Here's how the part is built. I have some questions about the finished solid (model axes, mm). A direction names the side the tool comes from. Coordinates: 2 decimals unless noted, no trailing zeros. Order: outer loops, then holes, each group sorted by start corner. A loop starts at its lowest first (then second) coordinate and runs counter-clockwise, first axis right, second up. Notation, with made-up numbers: (-13.75, -1) - (28.25, -1) arc R14 ccw to (28.25, 4) - close; hole circle Ø4 at (87.5, 15.5). An arc over 180 degrees is marked (long way). Answer as CSV lines item,"result". Start each with the question number.
Q1. Suppose I cut it at A-A (z = 47). Please give me the cut outline in (x, y), then the cut area to 3 significant figures.
Q2. I need wall thicknesses on line 1 (X direction, y = 21.75, z = 51); line 2 (Y direction, x = -56, z = 15); line 3 (Z direction, x = -5, y = 11.75). Which ranges of each line are inside material? Lowest first, please.
Q3. Thinking about a two-plate mould opening in Z: for faces 3 (the face through (2, 12, 5)), 4 (the face through (-23, 25, 72)), 5 (the face through (-27, 7, 75)), 6 (the face through (-57.487, 10.564, 17.307)), which applies, released by +Z, released by -Z, zero draft, split by the parting line, or undercut?
Q4. For faces 1 (the face through (-57.49, 22.15, 8.01)), 2 (the face through (-28, 7, 70)), which set-ups out of +Z, -Z, +X, -X, +Y, -Y let a thin tool reach every point of the face, with its end or its side?
Q5. For pin 1 Ø8 at (x, y) = (-6, 20) entering from -Z; pin 2 Ø2 at (y, z) = (15, 12) entering from -X, each with a flat end and sliding along its axis, tell me the tip position at first contact or that it passes through.
Q6. Suppose I cut it at B-B (z = 18). Please give me the cut outline in (x, y).
Q7. Suppose I cut it at D-D (x = -44). Please give me the cut outline in (y, z).
Q8. Suppose I cut it at C-C (y = 3). Please give me the cut outline in (x, z).
Autodesk Inventor part; units mm, degrees
ref_plane "YZ Plane" through (0, 0, 0) normal (1, 0, 0) x (0, 1, 0)
ref_plane "XZ Plane" through (0, 0, 0) normal (0, 1, 0) x (-1, 0, 0)
ref_plane "XY Plane" through (0, 0, 0) normal (0, 0, 1) x (1, 0, 0)
sketch "Sketch1" plane through (0, 0, 0) normal (0, 1, 0) x (-1, 0, 0)
  line L0 (0.1515, 5) -> (-4.8485, 5)
  line L1 (-4.8485, 5) -> (-4.8485, 75)
  line L2 (-4.8485, 75) -> (0.1515, 75)
  line L3 (0.1515, 75) -> (0.1515, 5)
  line L4 (54.9515, 5) -> (54.9515, 58.2)
  line L5 (54.9515, 5) -> (59.9515, 5)
  line L6 (59.9515, 5) -> (59.9515, 75)
  line L7 (59.9515, 75) -> (54.9515, 75)
  line L8 (54.9515, 75) -> (54.9515, 5)
  line L9 (0.1515, 75) -> (54.9515, 75)
  line L10 (54.9515, 75) -> (54.9515, 70)
  line L11 (54.9515, 70) -> (0.1515, 70)
  line L12 (0.1515, 70) -> (0.1515, 75)
  point P0 (0, 0)
  point P1 (55.2, 35)
  dimension "d0" = 5
  dimension "d1" = 70
  dimension "d2" = 5
  dimension "d3" = 5
  dimension "d10" = 54.8
extrude "Extrusion1" add sketch "Sketch1" along normal blind 25
fillet "Fillet1" radius 10 4 edges at (2.3485, 25, 5) (-57.4515, 25, 5) (2.3485, 0, 5) (-57.4515, 0, 5)
sketch "Sketch2" plane through (-59.9515, 0, 75) normal (-1, 0, 0) x (0, 0, 1)
  arc A0 (-60, 25) -> (-70, 15) centre (-60, 15) ccw
  circle A1 centre (-60, 15) radius 5
  point P0 (-75, 0)
  dimension "d7" = 10
extrude "Extrusion2" cut sketch "Sketch2" against normal blind 5
sketch "Sketch3" plane through (-0.1515, 0, 70) normal (-1, 0, 0) x (0, 0, 1)
  circle A0 centre (-55, 15) radius 5
  circle A1 centre (-55, 15) radius 5
  point P0 (-70, 0)
sketch "Sketch4" plane through (-59.9515, 0, 75) normal (0, 0, 1) x (1, 0, 0)
  circle A0 centre (32.4, 12.5) radius 4
  line L0 (0, 0) -> (64.8, 0)
  line L1 (0, 0) -> (0, 25)
  point P0 (59.9515, 0)
  dimension "d11" = 8
  dimension "d12" = 12.5
  dimension "d13" = 32.4
  dimension "d14" = 25
  dimension "d15" = 64.8
extrude "Extrusion3" cut sketch "Sketch4" against normal blind 5
properties part number "Hombro"
Here are the results:
1,outline,"(-59.95, 0) - (-54.95, 0) - (-54.95, 25) - (-59.95, 25) - close; (-0.15, 0) - (4.85, 0) - (4.85, 25) - (-0.15, 25) - close"
1,area,"250 mm²"
2,line 1,"x = -59.95 to -54.95, -0.15 to 4.85"
2,line 2,"y = 0 to 10, 20 to 25"
2,line 3,"z = 70 to 75"
3,face 3,"released by -Z"
3,face 4,"zero draft"
3,face 5,"released by +Z"
3,face 6,"undercut"
4,face 1,"-Z, +X, -X, +Y"
4,face 2,"-Z, +Y, -Y"
5,pin 1,"stops at z = 70"
5,pin 2,"stops at x = -0.15"
6,outline,"(-59.95, 0) - (-54.95, 0) - (-54.95, 11) - (-59.95, 11) - close; (-59.95, 19) - (-54.95, 19) - (-54.95, 25) - (-59.95, 25) - close; (-0.15, 0) - (4.85, 0) - (4.85, 25) - (-0.15, 25) - close"
7,outline,"(0, 70) - (25, 70) - (25, 75) - (0, 75) - close"
8,outline,"(-59.95, 7.86) - (-54.95, 7.86) - (-54.95, 70) - (-0.15, 70) - (-0.15, 7.86) - (4.85, 7.86) - (4.85, 75) - (-59.95, 75) - close"
